```python
from build123d import *

# Parameters (mm, degrees)
BOSS_EXTRUDE1_DEPTH = 12
CUT_EXTRUDE1_DEPTH  = 13.73


with BuildPart() as part:
    # Sketch1 → Boss-Extrude1 (new body)
    with BuildSketch(Plane(origin=(0, 0, 0), x_dir=(0, 0, -1), z_dir=(1, 0, 0))):
        Polygon((62.995348873, -5.73), (72.92, 0), (92.92, 0), (92.92, 3.314764861), (92.92, 8), (73.504568374, 8), (63.579917247, 2.27), (0, 2.27), (0, 0), (0, -5.73), (26.973026027, -5.73), align=None)
    extrude(amount=-BOSS_EXTRUDE1_DEPTH)

    # Sketch2 → Cut-Extrude1 (cut)
    with BuildSketch(Plane(origin=(0, 8, 0), x_dir=(1, 0, 0), z_dir=(0, 1, 0))):
        with BuildLine():
            ThreePointArc((-5.833418362, 12.299990394), (-10.32411062, 7.790701865), (-5.814822091, 3.300009606))
            Line((-5.814822091, 3.300009606), (-5.833418362, 12.299990394))
        make_face()
        with BuildLine():
            Line((-5.833418362, 12.299990394), (-5.814822091, 3.300009606))
            ThreePointArc((-5.814822091, 3.300009606), (-2.63885402, 4.621308572), (-1.324120226, 7.8))
            ThreePointArc((-1.324120226, 7.8), (-2.645428798, 10.985266206), (-5.833418362, 12.299990394))
        make_face()
        with BuildLine():
            ThreePointArc((-5.983738594, 85.0500168), (-8.478567627, 82.544856506), (-5.973407332, 80.050027474))
            Line((-5.973407332, 80.050027474), (-5.983738594, 85.0500168))
        make_face()
        with BuildLine():
            Line((-5.983738594, 85.0500168), (-5.973407332, 80.050027474))
            ThreePointArc((-5.973407332, 80.050027474), (-4.208980626, 80.784082455), (-3.478572963, 82.550022137))
            ThreePointArc((-3.478572963, 82.550022137), (-4.212633281, 84.319614474), (-5.983738594, 85.0500168))
        make_face()
    extrude(amount=-CUT_EXTRUDE1_DEPTH, mode=Mode.SUBTRACT)


solid = part.part
```
The model under review builds one solid part; all positions refer to its coordinate system, in mm. A direction names the side the tool comes from. Round coordinates to 2 decimals unless told otherwise and drop trailing zeros. Loops run counter-clockwise (first coordinate to the right, second up) from the corner with the lowest first, then second, coordinate; pieces in that order, holes last. Notation, with made-up numbers: (21.25, -6.5) -> (65.25, -6.5) arc R28 cw to (65.25, 22.5) -> close; hole circle Ø2 at (77.25, -34). An arc over 180 degrees is marked (long way). Answer in a Markdown table with one row per item.
1) For pin 1 Ø1 at (y, z) = (2.5, -54) entering from -X; pin 2 Ø3 at (x, y) = (-6, 4) entering from +Z; pin 3 Ø3.5 at (x, z) = (-6, -17.5) entering from +Y; pin 4 Ø3.5 at (x, z) = (-4.5, -80) entering from -Y, all flat-tipped, find the tip position at first contact; note any pin that passes through.
Taken from the geometry:
| item | result |
|---|---|
| pin 1 | stops at x = -12 |
| pin 2 | stops at z = -63.98 |
| pin 3 | stops at y = 2.27 |
| pin 4 | stops at y = 0 |
2) Consider section D-D, the plane z = -21. Write out the cut boundary in (x, y), plus the area to 3 significant figures.
Taken from the geometry:
| item | result |
|---|---|
| outline | (-12, -5.73) -> (0, -5.73) -> (0, 2.27) -> (-12, 2.27) -> close |
| area | 96.0 mm² |
3) Tool access review of faces 1 (the flat face through (-6, 4, -92.92)), 2 (the flat face through (-6, 2.27, -32)), 3 (the flat face through (-4.6, 0, -85)): name each direction out of +Z, -Z, +X, -X, +Y, -Y from which nothing blocks a thin tool from reaching the whole face with its end or side.
Taken from the geometry:
| item | result |
|---|---|
| face 1 | -Z, +X, -X, +Y, -Y |
| face 2 | +Z, +X, -X, +Y |
| face 3 | -Z, +X, -X, -Y |
4) Consider section B-B, the plane y = -3.25. Write out the cut boundary in (x, z).
Taken from the geometry:
| item | result |
|---|---|
| outline | (-12, -67.29) -> (0, -67.29) -> (0, 0) -> (-12, 0) -> close; hole circle Ø9 at (-5.82, -7.8) |
5) Consider section A-A, the plane x = -4.25. Write out the cut boundary in (y, z).
Taken from the geometry:
| item | result |
|---|---|
| outline | (-5.73, -63) -> (0, -72.92) -> (0, -80.74) -> (8, -80.74) -> (8, -73.5) -> (2.27, -63.58) -> (2.27, -12.02) -> (-5.73, -12.02) -> close; (-5.73, -3.58) -> (2.27, -3.58) -> (2.27, 0) -> (-5.73, 0) -> close; (0, -92.92) -> (8, -92.92) -> (8, -84.36) -> (0, -84.36) -> close |
6) Wall thickness on line 1 along Z through (x, y) = (-5.75, 1.75); line 2 along Z through (x, y) = (-4, 1); line 3 along Y through (x, z) = (-10.25, -5): over which ranges is each line inside the solid? List them lowest first.
Taken from the geometry:
| item | result |
|---|---|
| line 1 | z = -92.92 to -85.04, -80.06 to -12.3, -3.3 to 0 |
| line 2 | z = -92.92 to -84.08, -81.02 to -11.91, -3.69 to 0 |
| line 3 | y = -5.73 to 2.27 |
7) Consider section C-C, the plane y = 7. Write out the cut boundary in (x, z), plus the area to 3 significant figures.
Taken from the geometry:
| item | result |
|---|---|
| outline | (-12, -92.92) -> (0, -92.92) -> (0, -71.77) -> (-12, -71.77) -> close; hole circle Ø5 at (-5.98, -82.55) |
| area | 234 mm² |
